Can you work these out from the model? Positions are in its coordinate system, mm. A direction names the side the tool comes from. Coordinates: 2 decimals unless noted, no trailing zeros. Order: outer loops, then holes, each group sorted by start corner. A loop starts at its lowest first (then second) coordinate and runs counter-clockwise, first axis right, second up. Notation, with made-up numbers: M -12.75,38.25 L 31.25,38.25 A11 cw 31.25,54.25 Z; hole C 19,59 d6. An arc over 180 degrees is marked long. Answer as a JSON object with one key per item and string values.
from build123d import *

# Parameters (mm, degrees)
F_01_BASE_PROFILE_W           = 120
F_01_BASE_PROFILE_H           = 180
F_01_BASE_PROFILE_R           = 5.653846154
F_01_BASE_PROFILE_R_2         = 3.346153846
F_01_BASE_PROFILE_W_2         = 18
F_01_BASE_PROFILE_H_2         = 125
F_01_BASE_EXTRUDE_DEPTH       = 12
F_02_BOSS_PROFILE_W           = 82
F_02_BOSS_PROFILE_H           = 140
F_02_REINFORCEMENT_BOSS_DEPTH = 20


with BuildPart() as part:
    # 01_Base_Profile → 01_Base_Extrude (new body)
    with BuildSketch(Plane(origin=(0, 0, 0), x_dir=(1, 0, 0), z_dir=(0, 1, 0))):
        Rectangle(F_01_BASE_PROFILE_W, F_01_BASE_PROFILE_H)
        with Locations(Location((-46.153846154, -69.230769231, 0), (0, 0, 270))):
            Circle(F_01_BASE_PROFILE_R, mode=Mode.SUBTRACT)
        with Locations(Location((46.153846154, -69.230769231, 0), (0, 0, 270))):
            Circle(F_01_BASE_PROFILE_R_2, mode=Mode.SUBTRACT)
        with Locations(Location((-46.153846154, 69.230769231, 0), (0, 0, 270))):
            Circle(F_01_BASE_PROFILE_R, mode=Mode.SUBTRACT)
        with Locations(Location((46.153846154, 69.230769231, 0), (0, 0, 270))):
            Circle(F_01_BASE_PROFILE_R_2, mode=Mode.SUBTRACT)
        Rectangle(F_01_BASE_PROFILE_W_2, F_01_BASE_PROFILE_H_2, mode=Mode.SUBTRACT)
    extrude(amount=F_01_BASE_EXTRUDE_DEPTH)

    # 02_Boss_Profile → 02_Reinforcement_Boss (add)
    with BuildSketch(Plane(origin=(0, 0, 0), x_dir=(1, 0, 0), z_dir=(0, 1, 0))):
        Rectangle(F_02_BOSS_PROFILE_W, F_02_BOSS_PROFILE_H)
    extrude(amount=F_02_REINFORCEMENT_BOSS_DEPTH)


solid = part.part
Item 1: Which directions (+Z, -Z, +X, -X, +Y, -Y) give clear straight access to the entire face, cutting with the end or side of a thin tool? Please do faces 1 (the flat face through (41, 16, 1)), 2 (the flat face through (-1, 0, -1)).
Answers follow:
{"face 1": "+Z, -Z, +X, +Y", "face 2": "+Z, -Z, +X, -X, -Y"}
Item 2: I want a section at B-B, the plane z = -46.5. Write out the boundary of the cut face in (x, y).
Answers follow:
{"outline": "M -60,0 L 60,0 L 60,12 L 41,12 L 41,20 L -41,20 L -41,12 L -60,12 Z"}
Item 3: If we mould it in two halves opening along Z, with no side actions, what happens to faces 3 (the flat face through (60, 6, 1)), 4 (the cylindrical face through (-51.713, 5.916, -70.263)), 5 (the flat face through (-1, 6, -90))? For each: pulls with the +Z half, pulls with the -Z half, needs draft (parallel to the pull), parting line crosses it, or undercut.
Answers follow:
{"face 3": "needs draft", "face 4": "undercut", "face 5": "pulls with the -Z half"}
Item 4: I'm going to push flat-ended pins straight in: pin 1 (9 mm diameter, centred on x = -46.15, z = 69.23, fed in from +Y); pin 2 (7.5 mm diameter, centred on x = 46.15, z = 69.23, fed in from +Y); pin 3 (1 mm diameter, centred on y = 14.5, z = 16, fed in from +X); pin 4 (2 mm diameter, centred on x = 27.5, y = 14.5, fed in from +Z). Where does each tip first touch, or does it pass through?
Answers follow:
{"pin 1": "passes through", "pin 2": "stops at y = 12", "pin 3": "stops at x = 41", "pin 4": "stops at z = 70"}
Item 5: Please list where these lines run through material, in increasing order: line 1 (X direction, y = 19.25, z = -16.5); line 2 (Z direction, x = 29.5, y = 16.25); line 3 (Y direction, x = 15, z = 78.5).
Answers follow:
{"line 1": "x = -41 to 41", "line 2": "z = -70 to 70", "line 3": "y = 0 to 12"}
Item 6: I want a section at A-A, the plane x = 20.5. Write out the boundary of the cut face in (y, z), plus the area to 3 significant figures.
Answers follow:
{"outline": "M 0,-90 L 12,-90 L 12,-70 L 20,-70 L 20,70 L 12,70 L 12,90 L 0,90 Z", "area": "3,280 mm^2"}
Item 7: I want a section at C-C, the plane y = 17.5. Write out the boundary of the cut face in (x, z), plus the area to 3 significant figures.
Answers follow:
{"outline": "M -41,-70 L 41,-70 L 41,70 L -41,70 Z", "area": "11,500 mm^2"}
